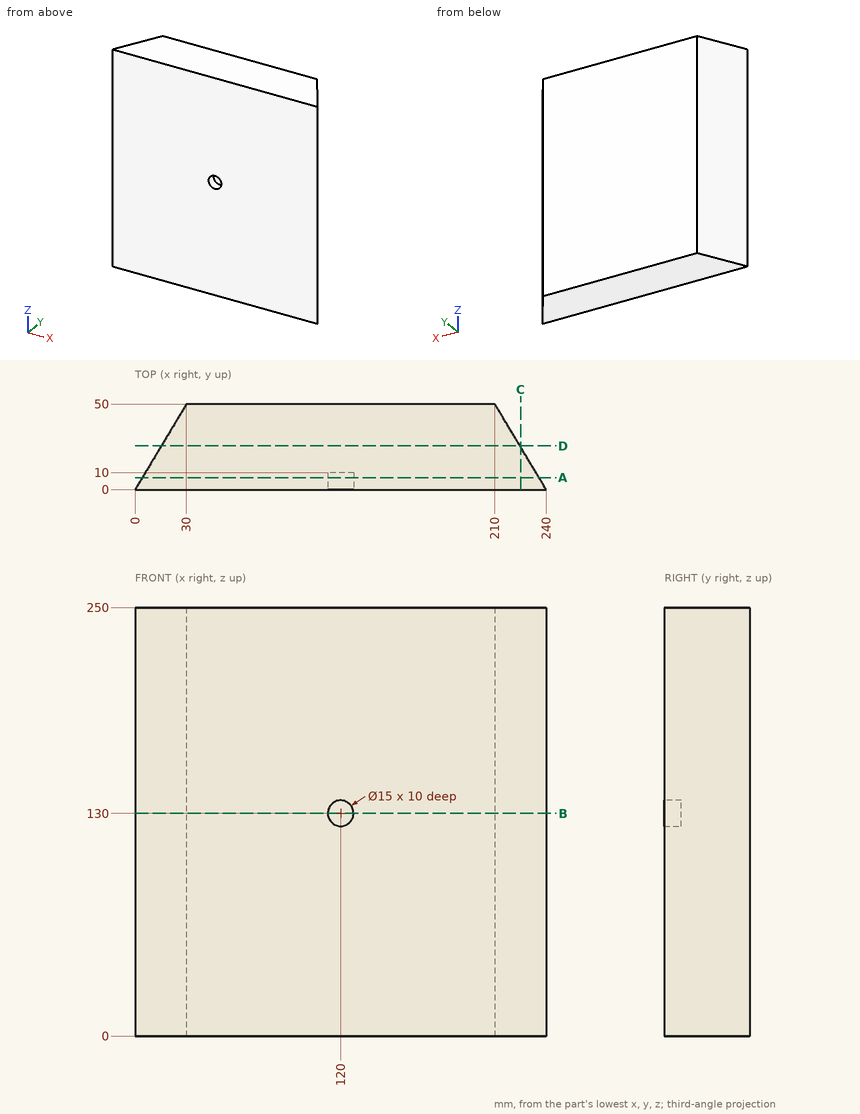
The figure shows three views and two pictorial views of one solid part (mm, origin at its lowest corner). Answer the questions. Give positions to 0.01 mm unless a question says otherwise; leave off trailing zeros. Order: outer loops, then holes, each group sorted by start corner. A loop starts at its lowest first (then second) coordinate and runs counter-clockwise, first axis right, second up. Notation, with made-up numbers: M 17,-37.75 L 68,-37.75 A30 ccw 68,1.25 Z; hole C 62,-27.75 d10. An arc over 180 degrees is marked long. Return JSON: item names as keys, results as strings.
1) Each of these flat-tipped pins is pushed along its axis until it touches: pin 1 (6 mm diameter, centred on y = 7.5, z = 75, fed in from -X); pin 2 (2 mm diameter, centred on y = 28.5, z = 161, fed in from +X). Where does it stop, or does it pass through?
Resolved:
{"pin 1": "x = 2.7", "pin 2": "x = 223.5"}
2) Section D-D, the plane y = 25.5 is taken. Write down the section's boundary in (x, z), plus the area to 4 significant figures.
Resolved:
{"outline": "M 15.3,0 L 224.7,0 L 224.7,250 L 15.3,250 Z", "area": "52,350 mm^2"}
3) Section A-A, the plane y = 7 is taken. Write down the section's boundary in (x, z), plus the area to 3 significant figures.
Resolved:
{"outline": "M 4.2,0 L 235.8,0 L 235.8,250 L 4.2,250 Z; hole C 120,130 d15", "area": "57,700 mm^2"}
4) Straight lines are drawn through the part: line 1 along X through (y, z) = (6, 130); line 2 along X through (y, z) = (3, 130); line 3 along Y through (x, z) = (13, 22). For each, find the intervals that lie inside material, in ascending order. Write a range as [from, to].
Resolved:
{"line 1": "[3.6, 112.5], [127.5, 236.4]", "line 2": "[1.8, 112.5], [127.5, 238.2]", "line 3": "[0, 21.67]"}
5) Section B-B, the plane z = 130 is taken. Write down the section's boundary in (x, y).
Resolved:
{"outline": "M 0,0 L 112.5,0 L 112.5,10 L 127.5,10 L 127.5,0 L 240,0 L 210,50 L 30,50 Z"}
6) Section C-C, the plane x = 225 is taken. Write down the section's boundary in (y, z), plus the area to 3 significant figures.
Resolved:
{"outline": "M 0,0 L 25,0 L 25,250 L 0,250 Z", "area": "6,250 mm^2"}
